The model under review builds one solid part; all positions refer to its coordinate system, in mm. Face numbers are marked on the shaded views. Round coordinates to 2 decimals unless told otherwise and drop trailing zeros. Write each loop counter-clockwise with the first axis right and the second up, starting at its lowest first coordinate (ties: lowest second). Pieces come first, ordered by that corner, then holes. Notation, with made-up numbers: (76.5, -1.75) -> (109.5, -1.75) arc R18 cw to (109.5, 6.25) -> close; hole circle Ø4 at (-18, -34.5). An arc over 180 degrees is marked (long way). Use CSV: the item, a comma, the result in double quotes. Start each with the question number.
1) Take a section at D-D, the plane z = 4.25. Give the boundary of the cut face in (x, y), then the cut area to 3 significant figures.
2) For pin 1 Ø1.5 at (y, z) = (-2, -1.5) entering from -X; pin 2 Ø0.5 at (y, z) = (0, -2.5) entering from -X; pin 3 Ø2 at (y, z) = (-3.5, 3.5) entering from +X; pin 4 Ø4 at (x, z) = (2, 3) entering from +Y, all flat-tipped, find the tip position at first contact; note any pin that passes through.
3) Mouldability with a two-part tool opening along Z and no side actions: class the marked faces 1, 2, 3 and 4 as released by +Z, released by -Z, zero draft, split by the parting line, or undercut.
4) Wall thickness on probe 1 along Z at (x, y) = (0, -2.45); probe 2 along X at (y, z) = (-0.4, -4.25); probe 3 along Z at (x, y) = (-1, -1.65): over which ranges is each line inside the solid? List them lowest first. Write a range as [from, to].
5) Take a section at B-B, the plane z = -3. Give the boundary of the cut face in (x, y), then the cut area to 3 significant figures.
6) Take a section at C-C, the plane y = -0.35. Give the boundary of the cut face in (x, z).
7) Take a section at A-A, the plane x = 0. Give the boundary of the cut face in (y, z).
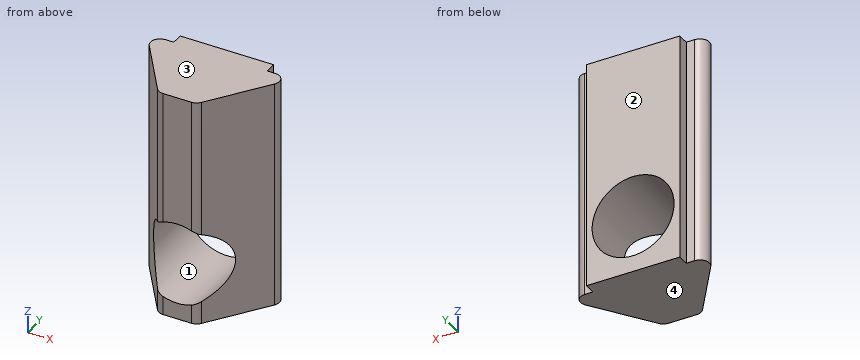
from build123d import *

# Parameters (mm, degrees)
BOSS_EXTRU_1_DEPTH      = 6
CONG_1_R                = 0.5
ENL_V_MAT_EXTRU_1_REACH = 10.281
ESQUISSE2_R             = 2.15


with BuildPart() as part:
    # Esquisse1 → Boss.-Extru.1 (new, symmetric)
    with BuildSketch(Plane.XY):
        Polygon((-2.45, 0), (2.45, 0), (2.45, -0.6), (3.85, -0.6), (1, -4.6), (-1, -4.6), (-3.85, -0.6), (-2.45, -0.6), align=None)
    extrude(amount=BOSS_EXTRU_1_DEPTH, both=True)

    # Congé1
    cong_1_edges = [part.edges().sort_by_distance(p)[0] for p in [
        (3.85, -0.6, 0),
        (1, -4.6, 0),
        (-1, -4.6, 0),
        (-3.85, -0.6, 0),
    ]]
    fillet(cong_1_edges, radius=CONG_1_R)

    # Esquisse2 → Enlèv. mat.-Extru.1 (cut, up to next)
    with BuildSketch(Plane(origin=(0, 0, 0), x_dir=(1, 0, 0), z_dir=(0, 1, 0)), mode=Mode.PRIVATE) as enl_v_mat_extru_1_sk1:
        with Locations(Location((0, 3, 0), (0, 0, 180))):
            Circle(ESQUISSE2_R)
    enl_v_mat_extru_1_tool1 = extrude(enl_v_mat_extru_1_sk1.sketch, amount=-ENL_V_MAT_EXTRU_1_REACH, mode=Mode.PRIVATE) & part.part
    add(enl_v_mat_extru_1_tool1.solids().sort_by_distance((0, 0, -3))[0], mode=Mode.SUBTRACT)


solid = part.part
Values found:
1,outline,"(-3.29, -1.39) -> (-1.15, -4.39) arc R0.5 ccw to (-0.74, -4.6) -> (0.74, -4.6) arc R0.5 ccw to (1.15, -4.39) -> (3.29, -1.39) arc R0.5 ccw to (2.88, -0.6) -> (2.45, -0.6) -> (2.45, 0) -> (-2.45, 0) -> (-2.45, -0.6) -> (-2.88, -0.6) arc R0.5 ccw to start"
1,area,"21.9 mm²"
2,pin 1,"x = -3.36"
2,pin 2,"x = -2.45"
2,pin 3,"x = 2.5"
2,pin 4,"y = 0"
3,face 1,"undercut"
3,face 2,"zero draft"
3,face 3,"released by +Z"
3,face 4,"released by -Z"
4,probe 1,"[-6, -5.15], [-0.85, 6]"
4,probe 2,"[-2.45, -1.75], [1.75, 2.45]"
4,probe 3,"[-6, -4.9], [-1.1, 6]"
5,outline,"(-3.29, -1.39) -> (-2.15, -2.99) -> (-2.15, 0) -> (-2.45, 0) -> (-2.45, -0.6) -> (-2.88, -0.6) arc R0.5 ccw to start; (2.15, -2.99) -> (3.29, -1.39) arc R0.5 ccw to (2.88, -0.6) -> (2.45, -0.6) -> (2.45, 0) -> (2.15, 0) -> close"
5,area,"3.99 mm²"
6,outline,"(-2.45, -6) -> (2.45, -6) -> (2.45, 6) -> (-2.45, 6) -> close; hole circle Ø4.3 at (0, -3)"
7,outline,"(-4.6, -6) -> (0, -6) -> (0, -5.15) -> (-4.6, -5.15) -> close; (-4.6, -0.85) -> (0, -0.85) -> (0, 6) -> (-4.6, 6) -> close"
